Source: CAD feature listing. Evaluate the final solid. Frame: model axes, mm. Face numbers are marked on the shaded views. A direction names the side the tool comes from. Give positions to 0.01 mm unless a question says otherwise; leave off trailing zeros. Loops run counter-clockwise (first coordinate to the right, second up) from the corner with the lowest first, then second, coordinate; pieces in that order, holes last. Notation, with made-up numbers: (-3, -16.75) - (5, -16.75) arc R16 ccw to (5, 7.25) - close; hole circle Ø2 at (67.25, 73.5). An arc over 180 degrees is marked (long way). Write each question's results on one line, items separated by ' | '. Start each with the question number.
(1) Cut plane B-B on z = -40.5. Return the cut outline in (x, y), then the cut area to 3 significant figures.
(2) Contact query for flat-ended pins moving along their axis: pin 1 (10 mm diameter, centred on x = -8, z = -74.5, fed in from +Y) (3 decimals); pin 2 (2 mm diameter, centred on x = 24, y = 9.5, fed in from -Z); pin 3 (4 mm diameter, centred on x = 60.5, y = 8.5, fed in from +Z). Output: stop coordinate, or through.
(3) Cut plane C-C on x = 32. Return the cut outline in (y, z).
(4) Pull-direction query (Z, two-part tool) for the marked faces 3, 4 and 5; classes: pulls with the +Z half, pulls with the -Z half, needs draft (parallel to the pull), parting line crosses it, or undercut.
(5) Material intervals for line 1 along Z through (x, y) = (57, 17); line 2 along X through (y, z) = (4.25, -104); line 3 along X through (y, z) = (2.75, -43), sorted ascending. Write a range as [from, to].
(6) Cut plane A-A on y = 11.5. Return the cut outline in (x, z), then the cut area to 3 significant figures.
(7) Reachability of the marked faces 1 and 2 from +Z, -Z, +X, -X, +Y, -Y: full face, straight path, thin tool, end or side. Return the list, or none.
from build123d import *

# Parameters (mm, degrees)
SKETCH1_W                = 101.092
SKETCH1_H                = 140.97
BOSS_EXTRUDE1_DEPTH      = 25.4
SKETCH2_W                = 100.076
SKETCH2_H                = 139.954
CUT_EXTRUDE1_DEPTH       = 21.336
SKETCH3_R                = 1.524
CUT_EXTRUDE2_DEPTH       = 21.336
SKETCH4_W                = 12.7
SKETCH4_H                = 3.175
BOSS_EXTRUDE2_DEPTH      = 12.7
F_5_16_18_TAPPED_HOLE1_D = 6.5278
SKETCH13_W               = 12.7
SKETCH13_H               = 3.175
BOSS_EXTRUDE3_DEPTH      = 12.7
F_5_16_18_TAPPED_HOLE2_D = 6.5278
FILLET1_R                = 7.62


with BuildPart() as part:
    # Sketch1 → Boss-Extrude1 (new body)
    with BuildSketch(Plane(origin=(0, 0, 0), x_dir=(1, 0, 0), z_dir=(0, 1, 0))):
        with Locations((50.546, 70.485)):
            Rectangle(SKETCH1_W, SKETCH1_H)
    extrude(amount=BOSS_EXTRUDE1_DEPTH)

    # Sketch2 → Cut-Extrude1 (cut)
    with BuildSketch(Plane(origin=(0, 25.4, 0), x_dir=(1, 0, 0), z_dir=(0, 1, 0))):
        with Locations((50.546, 70.485)):
            Rectangle(SKETCH2_W, SKETCH2_H)
    extrude(amount=-CUT_EXTRUDE1_DEPTH, mode=Mode.SUBTRACT)

    # Sketch3 → Cut-Extrude2 (cut)
    with BuildSketch(Plane(origin=(0, 4.064, 0), x_dir=(1, 0, 0), z_dir=(0, 1, 0))):
        with Locations((4.318, 136.525)):
            Circle(SKETCH3_R)
        with Locations((96.774, 136.525)):
            Circle(SKETCH3_R)
        with Locations((96.774, 4.191)):
            Circle(SKETCH3_R)
        with Locations((4.318, 4.191)):
            Circle(SKETCH3_R)
    extrude(amount=-CUT_EXTRUDE2_DEPTH, mode=Mode.SUBTRACT)

    # Sketch4 → Boss-Extrude2 (add)
    with BuildSketch(Plane(origin=(0, 0, -140.97), x_dir=(-1, 0, 0), z_dir=(0, 0, -1))):
        with Locations((-50.546, 1.5875)):
            Rectangle(SKETCH4_W, SKETCH4_H)
    boss_extrude2 = extrude(amount=BOSS_EXTRUDE2_DEPTH)

    # 5/16-18 Tapped Hole1 (through all)
    with Locations(Plane(origin=(0, 3.175, 0), x_dir=(1, 0, 0), z_dir=(0, 1, 0))):
        with Locations((50.546, 147.32)):
            f_5_16_18_tapped_hole1 = Hole(F_5_16_18_TAPPED_HOLE1_D / 2)

    # Mirror1: Boss-Extrude2, 5/16-18 Tapped Hole1 across plane
    add(boss_extrude2.mirror(Plane.XY.offset(-70.485)))
    add(f_5_16_18_tapped_hole1.mirror(Plane.XY.offset(-70.485)), mode=Mode.SUBTRACT)

    # Sketch13 → Boss-Extrude3 (add)
    with BuildSketch(Plane.ZY):
        with Locations((-70.485, 1.5875)):
            Rectangle(SKETCH13_W, SKETCH13_H)
    boss_extrude3 = extrude(amount=BOSS_EXTRUDE3_DEPTH)

    # 5/16-18 Tapped Hole2 (through all)
    with Locations(Plane(origin=(0, 3.175, 0), x_dir=(1, 0, 0), z_dir=(0, 1, 0))):
        with Locations((-6.35, 70.485)):
            f_5_16_18_tapped_hole2 = Hole(F_5_16_18_TAPPED_HOLE2_D / 2)

    # Mirror2: Boss-Extrude3, 5/16-18 Tapped Hole2 across plane
    add(boss_extrude3.mirror(Plane.ZY.offset(-50.546)))
    add(f_5_16_18_tapped_hole2.mirror(Plane.ZY.offset(-50.546)), mode=Mode.SUBTRACT)

    # Fillet1
    fillet1_edges = [part.edges().sort_by_distance(p)[0] for p in [
        (101.092, 1.5875, -64.135),
        (101.092, 1.5875, -76.835),
        (56.896, 1.5875, -140.97),
        (44.196, 1.5875, -140.97),
        (56.896, 1.5875, 0),
        (44.196, 1.5875, 0),
        (0, 1.5875, -64.135),
        (0, 1.5875, -76.835),
    ]]
    fillet(fillet1_edges, radius=FILLET1_R)


solid = part.part
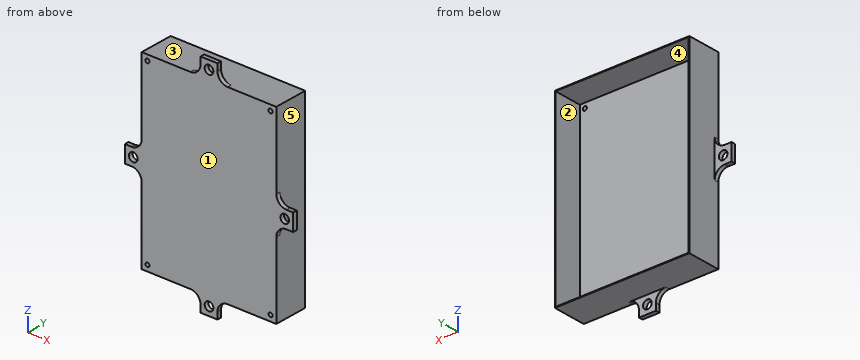
Ans:
1) outline: (0, 0) - (101.09, 0) - (101.09, 25.4) - (100.58, 25.4) - (100.58, 4.06) - (0.51, 4.06) - (0.51, 25.4) - (0, 25.4) - close | area: 433 mm^2
2) pin 1: y = 3.175 | pin 2: z = -140.97 | pin 3: z = 0
3) outline: (0, -140.97) - (25.4, -140.97) - (25.4, -140.46) - (4.06, -140.46) - (4.06, -0.51) - (25.4, -0.51) - (25.4, 0) - (0, 0) - close
4) face 3: pulls with the +Z half | face 4: undercut | face 5: needs draft
5) line 1: [-140.97, -140.46], [-0.51, 0] | line 2: [0, 0.51], [100.58, 101.09] | line 3: [0, 101.09]
6) outline: (0, -140.97) - (101.09, -140.97) - (101.09, 0) - (0, 0) - close; hole (0.51, -140.46) - (100.58, -140.46) - (100.58, -0.51) - (0.51, -0.51) - close | area: 245 mm^2
7) face 1: +Z, -Z, +X, -X, -Y | face 2: +Y
